Work out the finished part from the listing and answer in its coordinate system (mm). A direction names the side the tool comes from. Give positions to 0.01 mm unless a question says otherwise; leave off trailing zeros. Order: outer loops, then holes, each group sorted by start corner. A loop starts at its lowest first (then second) coordinate and runs counter-clockwise, first axis right, second up.
```python
from build123d import *

# Parameters (mm, degrees)
SKETCH1_W           = 150
SKETCH1_H           = 9
BOSS_EXTRUDE1_DEPTH = 6.5
SKETCH2_W           = 1
SKETCH2_H           = 1
CUT_EXTRUDE1_DEPTH  = 156.5
SKETCH3_R           = 1.8
CUT_EXTRUDE2_DEPTH  = 9.5
SKETCH4_R           = 3
CUT_EXTRUDE3_DEPTH  = 3.6
FILLET1_R           = 0.3
CHAMFER1_SIZE       = 0.3


with BuildPart() as part:
    # Sketch1 → Boss-Extrude1 (new body)
    with BuildSketch(Plane(origin=(0, 0, 0), x_dir=(1, 0, 0), z_dir=(0, 1, 0))):
        with Locations((75, 4.5)):
            Rectangle(SKETCH1_W, SKETCH1_H)
    extrude(amount=BOSS_EXTRUDE1_DEPTH)

    # Sketch2 → Cut-Extrude1 (cut)
    with BuildSketch(Plane(origin=(150, 0, 0), x_dir=(0, 0, -1), z_dir=(1, 0, 0))):
        with Locations((0.5, 5)):
            Rectangle(SKETCH2_W, SKETCH2_H)
        with Locations((8.5, 5)):
            Rectangle(SKETCH2_W, SKETCH2_H)
    extrude(amount=-CUT_EXTRUDE1_DEPTH, mode=Mode.SUBTRACT)

    # Sketch3 → Cut-Extrude2 (cut)
    with BuildSketch(Plane(origin=(0, 6.5, 0), x_dir=(1, 0, 0), z_dir=(0, 1, 0))):
        with Locations(Location((5, 4.5, 0), (0, 0, 270))):
            Circle(SKETCH3_R)
        with Locations(Location((25, 4.5, 0), (0, 0, 270))):
            Circle(SKETCH3_R)
        with Locations(Location((45, 4.5, 0), (0, 0, 270))):
            Circle(SKETCH3_R)
        with Locations(Location((65, 4.5, 0), (0, 0, 270))):
            Circle(SKETCH3_R)
        with Locations(Location((85, 4.5, 0), (0, 0, 270))):
            Circle(SKETCH3_R)
        with Locations(Location((105, 4.5, 0), (0, 0, 270))):
            Circle(SKETCH3_R)
        with Locations(Location((125, 4.5, 0), (0, 0, 270))):
            Circle(SKETCH3_R)
        with Locations(Location((145, 4.5, 0), (0, 0, 270))):
            Circle(SKETCH3_R)
    extrude(amount=-CUT_EXTRUDE2_DEPTH, mode=Mode.SUBTRACT)

    # Sketch4 → Cut-Extrude3 (cut)
    with BuildSketch(Plane(origin=(0, 6.5, 0), x_dir=(1, 0, 0), z_dir=(0, 1, 0))):
        with Locations(Location((5, 4.5, 0), (0, 0, 270))):
            Circle(SKETCH4_R)
        with Locations(Location((25, 4.5, 0), (0, 0, 270))):
            Circle(SKETCH4_R)
        with Locations(Location((45, 4.5, 0), (0, 0, 270))):
            Circle(SKETCH4_R)
        with Locations(Location((65, 4.5, 0), (0, 0, 270))):
            Circle(SKETCH4_R)
        with Locations(Location((85, 4.5, 0), (0, 0, 270))):
            Circle(SKETCH4_R)
        with Locations(Location((105, 4.5, 0), (0, 0, 270))):
            Circle(SKETCH4_R)
        with Locations(Location((125, 4.5, 0), (0, 0, 270))):
            Circle(SKETCH4_R)
        with Locations(Location((145, 4.5, 0), (0, 0, 270))):
            Circle(SKETCH4_R)
    extrude(amount=-CUT_EXTRUDE3_DEPTH, mode=Mode.SUBTRACT)

    # Fillet1
    fillet1_edges = [part.edges().sort_by_distance(p)[0] for p in [
        (75, 5.5, -1),
        (75, 4.5, -1),
        (75, 4.5, -8),
        (75, 5.5, -8),
    ]]
    fillet(fillet1_edges, radius=FILLET1_R)

    # Chamfer1
    chamfer1_edges = [part.edges().sort_by_distance(p)[0] for p in [
        (75, 5.5, -9),
        (75, 4.5, -9),
        (75, 6.5, -9),
        (75, 4.5, 0),
        (75, 5.5, 0),
        (75, 0, -9),
        (75, 0, 0),
        (75, 6.5, 0),
    ]]
    chamfer(chamfer1_edges, length=CHAMFER1_SIZE)


solid = part.part
```
1. Which of the six approach directions +Z, -Z, +X, -X, +Y, -Y give full straight-line access (tool end or side, diameter ignored) to faces 4 (the face through (150, 3, -4)), 5 (the face through (3, 2.9, -5))?
Findings below:
face 4: +Z, -Z, +X, +Y, -Y
face 5: +Y
2. The part is cut by section C-C (x = 34.5). Write down the section's boundary in (y, z).
Findings below:
outline: (0, -8.7) - (0.3, -9) - (4.2, -9) - (4.5, -8.7) - (4.5, -8.3) arc R0.3 cw to (4.8, -8) - (5.2, -8) arc R0.3 cw to (5.5, -8.3) - (5.5, -8.7) - (5.8, -9) - (6.2, -9) - (6.5, -8.7) - (6.5, -0.3) - (6.2, 0) - (5.8, 0) - (5.5, -0.3) - (5.5, -0.7) arc R0.3 cw to (5.2, -1) - (4.8, -1) arc R0.3 cw to (4.5, -0.7) - (4.5, -0.3) - (4.2, 0) - (0.3, 0) - (0, -0.3) - close
3. Given P1, Ø5, axis at x = 125, z = -4.5, coming from the +Y side, flat-ended and moving along its own axis, determine where the tip first touches the part or whether it passes through.
Findings below:
P1: stops at y = 2.9
4. The mould has two halves that part along Z. Classify faces 1 (the face through (74, 2, 0)), 2 (the face through (46.785, 1.47, -4.734)), 3 (the face through (0, 3, -4)): pulls with the +Z half, pulls with the -Z half, needs draft (parallel to the pull), parting line crosses it, or undercut.
Findings below:
face 1: pulls with the +Z half
face 2: undercut
face 3: needs draft
5. The part is cut by section A-A (y = 1.5). State how many separate pieces and enclosed holes the cut face has, then the cut area to 3 significant figures.
Findings below:
separate pieces: 1
enclosed holes: 8
area: 1,270 mm2
6. Straight lines are drawn through the part: probe 1 along Z at (x, y) = (105, 2.1); probe 2 along Y at (x, z) = (133, -8.25); probe 3 along Z at (x, y) = (101, 5). For each, find the intervals that lie inside material, in ascending order.
Findings below:
probe 1: z = -9 to -6.3, -2.7 to 0
probe 2: y = 0 to 4.5, 5.5 to 6.5
probe 3: z = -8 to -1
